Can you work these out from the model? Positions are in its coordinate system, mm. A direction names the side the tool comes from. Coordinates: 2 decimals unless noted, no trailing zeros. Write each loop counter-clockwise with the first axis right and the second up, starting at its lowest first coordinate (ties: lowest second). Pieces come first, ordered by that corner, then holes. Notation, with made-up numbers: M 89.25,37 L 93.25,37 A17 ccw 93.25,66 Z; hole C 79.5,64 d1. An arc over 180 degrees is marked long. Answer as a JSON object with one key per item and string values. Group by question number.
from build123d import *

# Parameters (mm, degrees)
SKETCH1_R             = 9.125
BOSS_EXTRUDE1_DEPTH   = 32.625
BOSS_EXTRUDE1_2_DEPTH = 32.625
BOSS_EXTRUDE1_3_DEPTH = 32.625
BOSS_EXTRUDE2_DEPTH   = 2.5
SKETCH3_W             = 37
SKETCH3_H             = 15
BOSS_EXTRUDE3_DEPTH   = 1.6
SKETCH4_R             = 0.775
BOSS_EXTRUDE4_DEPTH   = 8


with BuildPart() as part:
    # Sketch1 → Boss-Extrude1 (new, symmetric)
    with BuildSketch(Plane.XY):
        Circle(SKETCH1_R)
    extrude(amount=BOSS_EXTRUDE1_DEPTH, both=True)



with BuildPart() as body_2:
    # Sketch1 → Boss-Extrude1 2 (new, symmetric)
    with BuildSketch(Plane.XY):
        with Locations((18.575, 0)):
            Circle(SKETCH1_R)
    extrude(amount=BOSS_EXTRUDE1_2_DEPTH, both=True)


with BuildPart() as body_3:
    # Sketch1 → Boss-Extrude1 3 (new, symmetric)
    with BuildSketch(Plane.XY):
        with Locations((-18.575, 0)):
            Circle(SKETCH1_R)
    extrude(amount=BOSS_EXTRUDE1_3_DEPTH, both=True)


with BuildPart() as part_1:
    add(part.part)

    add(body_2.part)  # Boss-Extrude2 merges body 2

    add(body_3.part)  # Boss-Extrude2 merges body 3
    # Sketch2 → Boss-Extrude2 (add)
    with BuildSketch(Plane.XY.offset(32.625)):
        with BuildLine():
            Line((-18.575, 9.125), (18.575, 9.125))
            ThreePointArc((18.575, 9.125), (27.7, 0), (18.575, -9.125))
            Line((18.575, -9.125), (-18.575, -9.125))
            ThreePointArc((-18.575, -9.125), (-27.7, 0), (-18.575, 9.125))
        make_face()
    extrude(amount=BOSS_EXTRUDE2_DEPTH)

    # Sketch3 → Boss-Extrude3 (add)
    with BuildSketch(Plane.XY.offset(35.125)):
        Rectangle(SKETCH3_W, SKETCH3_H)
    extrude(amount=BOSS_EXTRUDE3_DEPTH)

    # Sketch4 → Boss-Extrude4 (add)
    with BuildSketch(Plane.XY.offset(35.125)):
        with Locations(Location((27.373251247, 2.42, 0), (0, 0, 107.8130031))):
            Circle(SKETCH4_R)
        with Locations(Location((27.373251247, -2.42, 0), (0, 0, 252.1869969))):
            Circle(SKETCH4_R)
    extrude(amount=BOSS_EXTRUDE4_DEPTH)


solid = part_1.part
Q1. Please list where these lines run through material, in increasing order: L1, parallel to X at y = 0.5, z = -28; L2, parallel to X at y = -7, z = 25; L3, parallel to Z at x = 0.5, y = -3.75 (3 decimals).
Q2. If we section it at A-A on y = 0: List the corners of the cut face in (x, z) for me (3 decimals), and give its area (3 significant figures).
Q3. On a 3-axis mill with a long thin cutter (end or side, diameter ignored), from which of +Z, -Z, +X, -X, +Y, -Y can I reach the whole of each face in a straight line? I mean faces 1 (the flat face through (0, -9.125, 34)), 2 (the flat face through (0, -7.5, 36)), 3 (the flat face through (9.3, -0.6, 32.625)). Say none if no direction works.
Q4. We'd pull the mould along Y, two halves only. Please class faces 4 (the flat face through (-18.5, 0, 36)), 5 (the flat face through (0, 7.5, 36)), 6 (the cylindrical face through (26.67, 2.09, 39.07)), 7 (the cylindrical face through (27.868, -3.017, 39.069)): pulls with the +Y half, pulls with the -Y half, needs draft (parallel to the pull), parting line crosses it, or undercut.
Q5. If we section it at B-B on x = 3: List the corners of the cut face in (y, z) for me (3 decimals).
Q6. If we section it at C-C on z = 9.5: List the corners of the cut face in (x, y) for me (3 decimals), and give its area (3 significant figures).
Q7. Will these pins go through, and if not, where does the flat tip stop? pin 1 (12 mm diameter, centred on x = -6, z = -4.5, fed in from +Y) (3 decimals); pin 2 (2 mm diameter, centred on x = -16, z = 24.5, fed in from -Y); pin 3 (0.8 mm diameter, centred on y = 0.5, z = 36, fed in from -X); pin 4 (8 mm diameter, centred on y = 5.5, z = 31, fed in from +X).
Q8. If we section it at D-D on y = 6: List the corners of the cut face in (x, z) for me (3 decimals).
Reply:
{
 "1": {"L1": "-27.69 to -9.46, -9.11 to 9.11, 9.46 to 27.69", "L2": "-24.43 to -12.72, -5.85 to 5.85, 12.72 to 24.43", "L3": "-32.625 to 36.725"},
 "2": {"outline": "M -27.7,-32.625 L -9.45,-32.625 L -9.45,32.625 L -9.125,32.625 L -9.125,-32.625 L 9.125,-32.625 L 9.125,32.625 L 9.45,32.625 L 9.45,-32.625 L 27.7,-32.625 L 27.7,35.125 L 18.5,35.125 L 18.5,36.725 L -18.5,36.725 L -18.5,35.125 L -27.7,35.125 Z", "area": "3,770 mm^2"},
 "3": {"face 1": "+Z, -Z, +X, -X, -Y", "face 2": "+Z, +X, -X, -Y", "face 3": "-Z"},
 "4": {"face 4": "needs draft", "face 5": "pulls with the +Y half", "face 6": "undercut", "face 7": "undercut"},
 "5": {"outline": "M -9.125,32.625 L -8.618,32.625 L -8.618,-32.625 L 8.618,-32.625 L 8.618,32.625 L 9.125,32.625 L 9.125,35.125 L 7.5,35.125 L 7.5,36.725 L -7.5,36.725 L -7.5,35.125 L -9.125,35.125 Z"},
 "6": {"outline": "C -18.575,0 d18.25; C 0,0 d18.25; C 18.575,0 d18.25", "area": "785 mm^2"},
 "7": {"pin 1": "y = 9.125", "pin 2": "y = -8.99", "pin 3": "x = -18.5", "pin 4": "x = 27.58"},
 "8": {"outline": "M -25.45,-32.625 L -11.7,-32.625 L -11.7,32.625 L -6.875,32.625 L -6.875,-32.625 L 6.875,-32.625 L 6.875,32.625 L 11.7,32.625 L 11.7,-32.625 L 25.45,-32.625 L 25.45,35.125 L 18.5,35.125 L 18.5,36.725 L -18.5,36.725 L -18.5,35.125 L -25.45,35.125 Z"}
}
